Work out the finished part from the listing and answer in its coordinate system (mm). A direction names the side the tool comes from. Coordinates: 2 decimals unless noted, no trailing zeros. Loops run counter-clockwise (first coordinate to the right, second up) from the corner with the lowest first, then second, coordinate; pieces in that order, holes last. Notation, with made-up numbers: (-28.75, -15) -> (-3.75, -15) arc R31 ccw to (-3.75, 23) -> close; hole circle Ø1 at (-31.75, 81.5). An arc over 180 degrees is marked (long way). Answer as CSV lines item,"result".
```python
from build123d import *

# Parameters (mm, degrees)
F1_DEPTH = 3
F2_W     = 20
F2_H     = 3
F2_W_2   = 24
F3_DEPTH = 3.001
F4_W     = 3
F4_H     = 20
F4_H_2   = 28
F5_DEPTH = 3.001
F6_R     = 3
F7_DEPTH = 3.001


with BuildPart() as f1:
    # F0 (on Front) → F1 (new body)
    with BuildSketch(Plane.XZ):
        Polygon((3, 3), (3, 0), (151, 0), (151, 3), (154, 3), (154, 111), (0, 111), (0, 3), align=None)
    extrude(amount=F1_DEPTH)

    # F2 (on face) → F3 (cut, through all)
    with BuildSketch(Plane.XZ.offset(3)):
        with Locations((13, 1.5)):
            Rectangle(F2_W, F2_H)
        with Locations((55, 1.5)):
            Rectangle(F2_W_2, F2_H)
        with Locations((141, 1.5)):
            Rectangle(F2_W, F2_H)
        with Locations((99, 1.5)):
            Rectangle(F2_W_2, F2_H)
    extrude(amount=-F3_DEPTH, mode=Mode.SUBTRACT)

    # F4 (on face) → F5 (cut, through all)
    with BuildSketch(Plane(origin=(0, 0, 0), x_dir=(-1, 0, 0), z_dir=(0, 1, 0))):
        with Locations((-152.5, 13)):
            Rectangle(F4_W, F4_H)
        with Locations((-152.5, 57)):
            Rectangle(F4_W, F4_H_2)
        with Locations((-152.5, 101)):
            Rectangle(F4_W, F4_H)
        with Locations((-1.5, 57)):
            Rectangle(F4_W, F4_H_2)
        with Locations((-1.5, 13)):
            Rectangle(F4_W, F4_H)
        with Locations((-1.5, 101)):
            Rectangle(F4_W, F4_H)
    extrude(amount=-F5_DEPTH, mode=Mode.SUBTRACT)

    # F6 (on face) → F7 (cut, through all)
    with BuildSketch(Plane(origin=(0, 0, 0), x_dir=(-1, 0, 0), z_dir=(0, 1, 0))):
        with Locations((-129, 19)):
            Circle(F6_R)
    extrude(amount=-F7_DEPTH, mode=Mode.SUBTRACT)


solid = f1.part
```
(1) For a pull along X with two mould halves and no side action, classify faces 5 (the face through (99, -2, 3)), 6 (the face through (131, -2, 1)), 7 (the face through (76, 0, 56)) as pulls with the +X half, pulls with the -X half, needs draft (parallel to the pull), parting line crosses it, or undercut.
Computed values:
face 5,"undercut"
face 6,"pulls with the +X half"
face 7,"needs draft"
(2) Flat-ended cylindrical pins translate along their axes: pin 1 Ø1.5 at (x, z) = (61, 13.5) entering from +Y; pin 2 Ø1.5 at (y, z) = (-1, 12) entering from -X; pin 3 Ø1.5 at (x, y) = (1.5, -1.5) entering from -Z; pin 4 Ø1.5 at (x, y) = (10.5, -2) entering from -Z. Find the tip coordinate at first contact, or state that the pin passes through.
Computed values:
pin 1,"y = 0"
pin 2,"x = 3"
pin 3,"z = 23"
pin 4,"z = 3"
(3) A cutting plane is placed at A-A, the plane x = 129. Write down the section's boundary in (y, z), and give its area (3 significant figures).
Computed values:
outline,"(-3, 0) -> (0, 0) -> (0, 16) -> (-3, 16) -> close; (-3, 22) -> (0, 22) -> (0, 111) -> (-3, 111) -> close"
area,"315 mm2"
(4) A cutting plane is placed at B-B, the plane z = 19. Write down the section's boundary in (x, y).
Computed values:
outline,"(3, -3) -> (126, -3) -> (126, 0) -> (3, 0) -> close; (132, -3) -> (151, -3) -> (151, 0) -> (132, 0) -> close"
(5) Consider line 1 along Z through (x, y) = (129, -0.8); line 2 along Z through (x, y) = (64.5, -0.55); line 3 along X through (y, z) = (-1.45, 63.5). Determine where each line is inside the solid, lowest interval first.
Computed values:
line 1,"0 to 16, 22 to 111"
line 2,"3 to 111"
line 3,"3 to 151"
(6) Which of the six approach directions +Z, -Z, +X, -X, +Y, -Y give full straight-line access (tool end or side, diameter ignored) to faces 1 (the face through (111, -2, 1)), 2 (the face through (153, -1, 91)), 3 (the face through (151, -1, 57)), 4 (the face through (2, -1, 43))?
Computed values:
face 1,"-Z, +Y, -Y"
face 2,"+Z, +X, +Y, -Y"
face 3,"+X, +Y, -Y"
face 4,"-X, +Y, -Y"
